```python
from build123d import *

# Parameters (mm, degrees)
SKETCH1_W           = 57
SKETCH1_H           = 57
BOSS_EXTRUDE1_DEPTH = 1.5
SKETCH2_R           = 28.5
BOSS_EXTRUDE2_DEPTH = 10
SKETCH3_R           = 27.5
BOSS_EXTRUDE3_DEPTH = 75
SKETCH4_R           = 28.5
BOSS_EXTRUDE4_DEPTH = 10
CUT_EXTRUDE1_REACH  = 127.739
SKETCH5_R           = 2.5
SKETCH6_R           = 19
BOSS_EXTRUDE5_DEPTH = 1.5
SKETCH7_R           = 4
BOSS_EXTRUDE6_DEPTH = 20
FILLET1_R           = 5
FILLET2_R           = 0.5


with BuildPart() as part:
    # Sketch1 → Boss-Extrude1 (new body)
    with BuildSketch(Plane.XY):
        with Locations((28.5, 28.5)):
            Rectangle(SKETCH1_W, SKETCH1_H)
    extrude(amount=BOSS_EXTRUDE1_DEPTH)

    # Sketch2 → Boss-Extrude2 (add)
    with BuildSketch(Plane.XY.offset(1.5)):
        with Locations((28.5, 28.5)):
            Circle(SKETCH2_R)
    extrude(amount=BOSS_EXTRUDE2_DEPTH)

    # Sketch3 → Boss-Extrude3 (add)
    with BuildSketch(Plane.XY.offset(11.5)):
        with Locations((28.5, 28.5)):
            Circle(SKETCH3_R)
    extrude(amount=BOSS_EXTRUDE3_DEPTH)

    # Sketch4 → Boss-Extrude4 (add)
    with BuildSketch(Plane.XY.offset(86.5)):
        with Locations((28.5, 28.5)):
            Circle(SKETCH4_R)
    extrude(amount=BOSS_EXTRUDE4_DEPTH)

    # Sketch5 → Cut-Extrude1 (cut, up to next)
    with BuildSketch(Plane(origin=(0, 0, 0), x_dir=(-1, 0, 0), z_dir=(0, 0, -1)), mode=Mode.PRIVATE) as cut_extrude1_sk1:
        with Locations((-52, 52)):
            Circle(SKETCH5_R)
    cut_extrude1_tool1 = extrude(cut_extrude1_sk1.sketch, amount=-CUT_EXTRUDE1_REACH, mode=Mode.PRIVATE) & part.part
    # Sketch5 → Cut-Extrude1 (cut, up to next)
    with BuildSketch(Plane(origin=(0, 0, 0), x_dir=(-1, 0, 0), z_dir=(0, 0, -1)), mode=Mode.PRIVATE) as cut_extrude1_sk2:
        with Locations((-5, 52)):
            Circle(SKETCH5_R)
    cut_extrude1_tool2 = extrude(cut_extrude1_sk2.sketch, amount=-CUT_EXTRUDE1_REACH, mode=Mode.PRIVATE) & part.part
    # Sketch5 → Cut-Extrude1 (cut, up to next)
    with BuildSketch(Plane(origin=(0, 0, 0), x_dir=(-1, 0, 0), z_dir=(0, 0, -1)), mode=Mode.PRIVATE) as cut_extrude1_sk3:
        with Locations((-5, 5)):
            Circle(SKETCH5_R)
    cut_extrude1_tool3 = extrude(cut_extrude1_sk3.sketch, amount=-CUT_EXTRUDE1_REACH, mode=Mode.PRIVATE) & part.part
    # Sketch5 → Cut-Extrude1 (cut, up to next)
    with BuildSketch(Plane(origin=(0, 0, 0), x_dir=(-1, 0, 0), z_dir=(0, 0, -1)), mode=Mode.PRIVATE) as cut_extrude1_sk4:
        with Locations((-52, 5)):
            Circle(SKETCH5_R)
    cut_extrude1_tool4 = extrude(cut_extrude1_sk4.sketch, amount=-CUT_EXTRUDE1_REACH, mode=Mode.PRIVATE) & part.part
    add(cut_extrude1_tool1.solids().sort_by_distance((52, 52, 0))[0], mode=Mode.SUBTRACT)
    add(cut_extrude1_tool2.solids().sort_by_distance((5, 52, 0))[0], mode=Mode.SUBTRACT)
    add(cut_extrude1_tool3.solids().sort_by_distance((5, 5, 0))[0], mode=Mode.SUBTRACT)
    add(cut_extrude1_tool4.solids().sort_by_distance((52, 5, 0))[0], mode=Mode.SUBTRACT)

    # Sketch6 → Boss-Extrude5 (add)
    with BuildSketch(Plane(origin=(0, 0, 0), x_dir=(-1, 0, 0), z_dir=(0, 0, -1))):
        with Locations(Location((-28.5, 28.5, 0), (0, 0, 180))):
            Circle(SKETCH6_R)
    extrude(amount=BOSS_EXTRUDE5_DEPTH)

    # Sketch7 → Boss-Extrude6 (add)
    with BuildSketch(Plane(origin=(0, 0, -1.5), x_dir=(-1, 0, 0), z_dir=(0, 0, -1))):
        with Locations((-28.5, 28.5)):
            Circle(SKETCH7_R)
    extrude(amount=BOSS_EXTRUDE6_DEPTH)

    # Fillet1
    fillet1_edges = [part.edges().sort_by_distance(p)[0] for p in [
        (0, 57, 0.75),
        (57, 57, 0.75),
        (57, 0, 0.75),
        (0, 0, 0.75),
    ]]
    fillet(fillet1_edges, radius=FILLET1_R)

    # Fillet2
    fillet2_edges = [part.edges().sort_by_distance(p)[0] for p in [
        (1, 28.5, 11.5),
        (1, 28.5, 86.5),
        (0, 28.5, 96.5),
        (9.5, 28.5, 0),
        (9.5, 28.5, -1.5),
    ]]
    fillet(fillet2_edges, radius=FILLET2_R)


solid = part.part
```
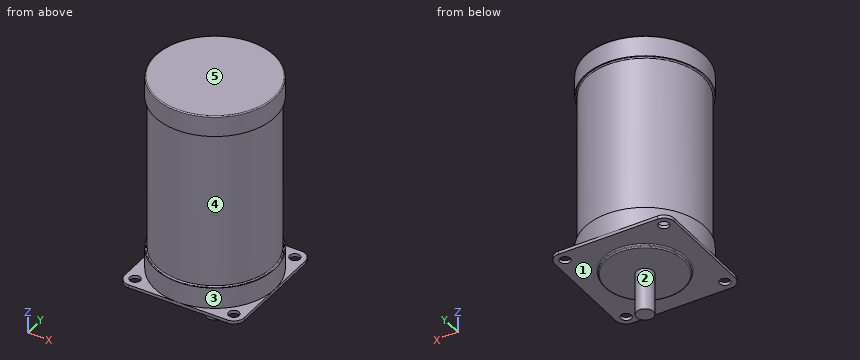
The model under review builds one solid part; all positions refer to its coordinate system, in mm. Face numbers are marked on the shaded views. A direction names the side the tool comes from. Coordinates: 2 decimals unless noted, no trailing zeros. Write each loop counter-clockwise with the first axis right and the second up, starting at its lowest first coordinate (ties: lowest second). Pieces come first, ordered by that corner, then holes.
1) We need section B-B on z = 36. State the section outline as (x, y) points.
2) We need section A-A on z = 3.5. State the section outline as (x, y) points, then the cut area to 3 significant figures.
3) Clearance check with flat-ended pins moving along their axes: pin 1 Ø1.5 at (y, z) = (30.5, -1.5) entering from +X; pin 2 Ø12 at (x, y) = (51, 9.5) entering from -Z; pin 3 Ø17 at (x, y) = (36.5, 18) entering from -Z. State where each tip first meets the part, or that it passes through.
4) Machinability: for the marked faces 3, 4 and 5, which of the approach directions +Z, -Z, +X, -X, +Y, -Y give a long, thin tool a straight path to every point of the face, cutting with its end or side? Answer none if there is none.
5) To check wall thickness, follow probe 1 along Y at (x, z) = (5, 0.8); probe 2 along Z at (x, y) = (27, 18); probe 3 along X at (y, z) = (6, 1). State the ranges of each line that lie inside material, in increasing order.
6) The part is to be moulded in two halves that separate along X. For the marked faces 1 and 2, say which applies: pulls with the +X half, pulls with the -X half, needs draft (parallel to the pull), parting line crosses it, or undercut.
Answer list:
1. outline: circle Ø55 at (28.5, 28.5)
2. outline: circle Ø57 at (28.5, 28.5)
2. area: 2,550 mm2
3. pin 1: stops at x = 47.45
3. pin 2: stops at z = 0
3. pin 3: stops at z = -1.5
4. face 3: +Z
4. face 4: none
4. face 5: +Z, +X, -X, +Y, -Y
5. probe 1: y = 0 to 2.5, 7.5 to 49.5, 54.5 to 57
5. probe 2: z = -1.5 to 96.5
5. probe 3: x = 0 to 2.71, 7.29 to 49.71, 54.29 to 57
6. face 1: needs draft
6. face 2: parting line crosses it
